Work out the finished part from the listing and answer in its coordinate system (mm). A direction names the side the tool comes from. Give positions to 0.01 mm unless a question says otherwise; leave off trailing zeros. Loops run counter-clockwise (first coordinate to the right, second up) from the corner with the lowest first, then second, coordinate; pieces in that order, holes last. Notation, with made-up numbers: (48, -10) - (61, -10) arc R15 cw to (61, -6) - close; hole circle Ø4 at (49, 73.25). An arc over 180 degrees is marked (long way). One line per question, with ' | ' between items.
from build123d import *

# Parameters (mm, degrees)
F4_DEPTH  = 3.175
F5_DEPTH  = 25.4
F6_R      = 3.1
F6_R_2    = 2.54
F6_W      = 19.05
F6_H      = 3.175
F0_R      = 3.1
F0_R_2    = 1.375
F7_DEPTH  = 3.175
F8_R      = 1.27
F9_DEPTH  = 5.08
F10_R     = 3.048
F11_DEPTH = 3.175
F12_R     = 3.96875
F13_DEPTH = 97.276
F15_DEPTH = 3.175
F16_R     = 2.921
F16_R_2   = 2.54
F17_DEPTH = 3.175
F18_R     = 2.54
F19_R     = 5.08
F19_R_2   = 1.5875
F20_DEPTH = 25.4


with BuildPart() as f4:
    # F3 (on Top) → F4 (new body)
    with BuildSketch(Plane.XY):
        Polygon((-26.1401280605, 113.175), (-34.35, 104.9651280605), (-34.35, -36.6401280605), (-26.1401280605, -44.85), (54.7151280605, -44.85), (62.925, -36.6401280605), (62.925, 104.9651280605), (54.7151280605, 113.175), align=None)
        Polygon((-31.175, 103.65), (-24.825, 110), (53.4, 110), (59.75, 103.65), (59.75, -35.325), (53.4, -41.675), (-24.825, -41.675), (-31.175, -35.325), align=None, mode=Mode.SUBTRACT)
        Polygon((53.4, 110), (-24.825, 110), (-31.175, 103.65), (-31.175, -35.325), (-24.825, -41.675), (53.4, -41.675), (59.75, -35.325), (59.75, 103.65), align=None)
    extrude(amount=-F4_DEPTH)

    # F3 (on Top) → F5 (join)
    with BuildSketch(Plane.XY):
        Polygon((-26.1401280605, 113.175), (-34.35, 104.9651280605), (-34.35, -36.6401280605), (-26.1401280605, -44.85), (54.7151280605, -44.85), (62.925, -36.6401280605), (62.925, 104.9651280605), (54.7151280605, 113.175), align=None)
        Polygon((-31.175, 103.65), (-24.825, 110), (53.4, 110), (59.75, 103.65), (59.75, -35.325), (53.4, -41.675), (-24.825, -41.675), (-31.175, -35.325), align=None, mode=Mode.SUBTRACT)
    extrude(amount=F5_DEPTH)

    # F6 (on face) + F0 (on Top) → F7 (join)
    with BuildSketch(Plane.XY):
        with Locations((-24.5, 23)):
            Circle(F6_R)
        with Locations((24.5, 23)):
            Circle(F6_R)
        with Locations((-24.5, -35)):
            Circle(F6_R)
        with Locations((24.5, -35)):
            Circle(F6_R)
        with Locations((33.715, 43.96)):
            Circle(F6_R_2)
        with Locations((48.955, 43.96)):
            Circle(F6_R_2)
        with Locations((33.715, 22.37)):
            Circle(F6_R_2)
        with Locations((48.955, 22.37)):
            Circle(F6_R_2)
        with Locations((33.715, -0.654)):
            Circle(F6_R_2)
        with Locations((54.035, -0.654)):
            Circle(F6_R_2)
        with Locations((43.875, -30.5625)):
            Rectangle(F6_W, F6_H)
    with BuildSketch(Plane.XY):
        with Locations((-24.5, 23)):
            Circle(F0_R)
        with Locations((-24.5, 23)):
            Circle(F0_R_2, mode=Mode.SUBTRACT)
    extrude(amount=F7_DEPTH)

    # F8 (on face) → F9 (cut)
    with BuildSketch(Plane.XY.offset(3.175)):
        with Locations((-24.5, 23)):
            Circle(F8_R)
        with Locations((24.5, 23)):
            Circle(F8_R)
        with Locations((24.5, -35)):
            Circle(F8_R)
        with Locations((-24.5, -35)):
            Circle(F8_R)
        with Locations((33.715, 43.96)):
            Circle(F8_R)
        with Locations((48.955, 43.96)):
            Circle(F8_R)
        with Locations((33.715, 22.37)):
            Circle(F8_R)
        with Locations((48.955, 22.37)):
            Circle(F8_R)
        with Locations((33.715, -0.654)):
            Circle(F8_R)
        with Locations((54.035, -0.654)):
            Circle(F8_R)
    extrude(amount=-F9_DEPTH, mode=Mode.SUBTRACT)

    # F10 (on face) → F11 (cut, through all)
    with BuildSketch(Plane(origin=(-34.35, 0, 0), x_dir=(0, -1, 0), z_dir=(-1, 0, 0))):
        with Locations((27.2421280605, 19.812)):
            Circle(F10_R)
    extrude(amount=-F11_DEPTH, mode=Mode.SUBTRACT)

    # F12 (on face) → F13 (cut, through all)
    with BuildSketch(Plane(origin=(-34.35, 0, 0), x_dir=(0, -1, 0), z_dir=(-1, 0, 0))):
        with Locations((-94.6463780605, 15.08125)):
            Circle(F12_R)
    extrude(amount=-F13_DEPTH, mode=Mode.SUBTRACT)

    # F14 (on face) → F15 (cut, through all)
    with BuildSketch(Plane(origin=(0, 113.175, 0), x_dir=(-1, 0, 0), z_dir=(0, 1, 0))):
        with BuildLine():
            Line((-19.3675, 20.32), (-20.6375, 20.32))
            ThreePointArc((-20.6375, 20.32), (-21.5355256121, 19.9480256121), (-21.9075, 19.05))
            Line((-21.9075, 19.05), (-21.9075, 6.35))
            ThreePointArc((-21.9075, 6.35), (-21.5355256121, 5.4519743879), (-20.6375, 5.08))
            Line((-20.6375, 5.08), (-19.3675, 5.08))
            ThreePointArc((-19.3675, 5.08), (-18.4694743879, 5.4519743879), (-18.0975, 6.35))
            Line((-18.0975, 6.35), (-18.0975, 19.05))
            ThreePointArc((-18.0975, 19.05), (-18.4694743879, 19.9480256121), (-19.3675, 20.32))
        make_face()
        with BuildLine():
            Line((-25.7175, 6.35), (-25.7175, 19.05))
            ThreePointArc((-25.7175, 19.05), (-26.0894743879, 19.9480256121), (-26.9875, 20.32))
            Line((-26.9875, 20.32), (-28.2575, 20.32))
            ThreePointArc((-28.2575, 20.32), (-29.1555256121, 19.9480256121), (-29.5275, 19.05))
            Line((-29.5275, 19.05), (-29.5275, 6.35))
            ThreePointArc((-29.5275, 6.35), (-29.1555256121, 5.4519743879), (-28.2575, 5.08))
            Line((-28.2575, 5.08), (-26.9875, 5.08))
            ThreePointArc((-26.9875, 5.08), (-26.0894743879, 5.4519743879), (-25.7175, 6.35))
        make_face()
        with BuildLine():
            Line((-33.3375, 6.35), (-33.3375, 19.05))
            ThreePointArc((-33.3375, 19.05), (-33.7094743879, 19.9480256121), (-34.6075, 20.32))
            Line((-34.6075, 20.32), (-35.8775, 20.32))
            ThreePointArc((-35.8775, 20.32), (-36.7755256121, 19.9480256121), (-37.1475, 19.05))
            Line((-37.1475, 19.05), (-37.1475, 6.35))
            ThreePointArc((-37.1475, 6.35), (-36.7755256121, 5.4519743879), (-35.8775, 5.08))
            Line((-35.8775, 5.08), (-34.6075, 5.08))
            ThreePointArc((-34.6075, 5.08), (-33.7094743879, 5.4519743879), (-33.3375, 6.35))
        make_face()
        with BuildLine():
            Line((-40.9575, 6.35), (-40.9575, 19.05))
            ThreePointArc((-40.9575, 19.05), (-41.3294743879, 19.9480256121), (-42.2275, 20.32))
            Line((-42.2275, 20.32), (-43.4975, 20.32))
            ThreePointArc((-43.4975, 20.32), (-44.3955256121, 19.9480256121), (-44.7675, 19.05))
            Line((-44.7675, 19.05), (-44.7675, 6.35))
            ThreePointArc((-44.7675, 6.35), (-44.3955256121, 5.4519743879), (-43.4975, 5.08))
            Line((-43.4975, 5.08), (-42.2275, 5.08))
            ThreePointArc((-42.2275, 5.08), (-41.3294743879, 5.4519743879), (-40.9575, 6.35))
        make_face()
        with BuildLine():
            Line((-7.9375, 19.9480256121), (-9.2075, 19.9480256121))
            ThreePointArc((-9.2075, 19.9480256121), (-10.1055256121, 19.5760512242), (-10.4775, 18.6780256121))
            Line((-10.4775, 18.6780256121), (-10.4775, 6.35))
            ThreePointArc((-10.4775, 6.35), (-10.1055256121, 5.4519743879), (-9.2075, 5.08))
            Line((-9.2075, 5.08), (-7.9375, 5.08))
            ThreePointArc((-7.9375, 5.08), (-7.0394743879, 5.4519743879), (-6.6675, 6.35))
            Line((-6.6675, 6.35), (-6.6675, 18.6780256121))
            ThreePointArc((-6.6675, 18.6780256121), (-7.0394743879, 19.5760512242), (-7.9375, 19.9480256121))
        make_face()
        with BuildLine():
            ThreePointArc((-1.5875, 19.9480256121), (-2.4855256121, 19.5760512242), (-2.8575, 18.6780256121))
            Line((-2.8575, 18.6780256121), (-2.8575, 6.35))
            ThreePointArc((-2.8575, 6.35), (-2.4855256121, 5.4519743879), (-1.5875, 5.08))
            Line((-1.5875, 5.08), (-0.3175, 5.08))
            ThreePointArc((-0.3175, 5.08), (0.5805256121, 5.4519743879), (0.9525, 6.35))
            Line((0.9525, 6.35), (0.9525, 18.6780256121))
            ThreePointArc((0.9525, 18.6780256121), (0.5805256121, 19.5760512242), (-0.3175, 19.9480256121))
            Line((-0.3175, 19.9480256121), (-1.5875, 19.9480256121))
        make_face()
        with BuildLine():
            ThreePointArc((6.0325, 19.9480256121), (5.1344743879, 19.5760512242), (4.7625, 18.6780256121))
            Line((4.7625, 18.6780256121), (4.7625, 6.35))
            ThreePointArc((4.7625, 6.35), (5.1344743879, 5.4519743879), (6.0325, 5.08))
            Line((6.0325, 5.08), (7.3025, 5.08))
            ThreePointArc((7.3025, 5.08), (8.2005256121, 5.4519743879), (8.5725, 6.35))
            Line((8.5725, 6.35), (8.5725, 18.6780256121))
            ThreePointArc((8.5725, 18.6780256121), (8.2005256121, 19.5760512242), (7.3025, 19.9480256121))
            Line((7.3025, 19.9480256121), (6.0325, 19.9480256121))
        make_face()
        with BuildLine():
            ThreePointArc((13.6525, 19.9480256121), (12.7544743879, 19.5760512242), (12.3825, 18.6780256121))
            Line((12.3825, 18.6780256121), (12.3825, 6.35))
            ThreePointArc((12.3825, 6.35), (12.7544743879, 5.4519743879), (13.6525, 5.08))
            Line((13.6525, 5.08), (14.9225, 5.08))
            ThreePointArc((14.9225, 5.08), (15.8205256121, 5.4519743879), (16.1925, 6.35))
            Line((16.1925, 6.35), (16.1925, 18.6780256121))
            ThreePointArc((16.1925, 18.6780256121), (15.8205256121, 19.5760512242), (14.9225, 19.9480256121))
            Line((14.9225, 19.9480256121), (13.6525, 19.9480256121))
        make_face()
    extrude(amount=-F15_DEPTH, mode=Mode.SUBTRACT)

    # F16 (on face) → F17 (cut, through all)
    with BuildSketch(Plane.XZ.offset(44.85)):
        with Locations((-16.8691280605, 19.304)):
            Circle(F16_R)
        with Locations((-4.1691280605, 19.304)):
            Circle(F16_R)
        with Locations((8.5308719395, 19.304)):
            Circle(F16_R)
        with Locations((21.2308719395, 19.304)):
            Circle(F16_R_2)
    extrude(amount=-F17_DEPTH, mode=Mode.SUBTRACT)

    # F18
    f18_edges = [f4.edges().sort_by_distance(p)[0] for p in [
        (62.925, -36.640128, 11.1125),
        (54.715128, -44.85, 11.1125),
        (62.925, 104.965128, 11.1125),
        (54.715128, 113.175, 11.1125),
        (-26.140128, 113.175, 11.1125),
        (-34.35, 104.965128, 11.1125),
        (-34.35, -36.640128, 11.1125),
        (-26.140128, -44.85, 11.1125),
    ]]
    fillet(f18_edges, radius=F18_R)

    # F19 (on face) → F20 (join)
    with BuildSketch(Plane.XY):
        with Locations((-5.775, 89.68)):
            Circle(F19_R)
        with Locations((-5.775, 89.68)):
            Circle(F19_R_2, mode=Mode.SUBTRACT)
        with Locations((29.27, 89.68)):
            Circle(F19_R)
        with Locations((29.27, 89.68)):
            Circle(F19_R_2, mode=Mode.SUBTRACT)
        with Locations((41.97, 10.94)):
            Circle(F19_R)
        with Locations((41.97, 10.94)):
            Circle(F19_R_2, mode=Mode.SUBTRACT)
    extrude(amount=F20_DEPTH)


solid = f4.part
1. Consider L1, parallel to Y at x = 13.5, z = 18 (3 decimals); L2, parallel to X at y = -17, z = 9 (3 decimals); L3, parallel to Y at x = 46.5, z = 17.25 (3 decimals). Determine where each line is inside the solid, lowest interval first.
Evaluation:
L1: -44.85 to -41.675, 110 to 113.175 | L2: -34.35 to -31.175, 59.75 to 62.925 | L3: -44.85 to -41.675, 8.641 to 13.239, 110 to 113.175
2. Find section A-A on y = 66. Write down the section's boundary in (x, z) (3 decimals).
Evaluation:
outline: (-34.35, -3.175) - (62.925, -3.175) - (62.925, 25.4) - (59.75, 25.4) - (59.75, 0) - (-31.175, 0) - (-31.175, 25.4) - (-34.35, 25.4) - close
3. Which of the six approach directions +Z, -Z, +X, -X, +Y, -Y give full straight-line access (tool end or side, diameter ignored) to faces 1 (the cylindrical face through (20.9, -43.285, 21.822)), 2 (the flat face through (21.908, 112, 13)), 3 (the flat face through (34, 24, 3.175))?
Evaluation:
face 1: -Y | face 2: +Y | face 3: +Z
4. Flat-ended cylindrical pins translate along their axes: pin 1 (3 mm diameter, centred on x = 48.955, y = 22.37, fed in from +Z) (3 decimals); pin 2 (3 mm diameter, centred on x = 0.5, y = 36.5, fed in from +Z); pin 3 (1.6 mm diameter, centred on y = 112, z = 10.5, fed in from -X). Find the tip coordinate at first contact, or state that the pin passes through.
Evaluation:
pin 1: z = 3.175 | pin 2: z = 0 | pin 3: x = -28.12
5. Determine the mould class of faces 4 (the flat face through (18.098, 112, 13)), 5 (the flat face through (34, 1, 3.175)), 6 (the cylindrical face through (-24.904, -31.926, 1.565)) for opening direction Z: +Z half, -Z half, draft (parallel to the pull), parting line (faces both ways), or undercut.
Evaluation:
face 4: undercut | face 5: +Z half | face 6: draft
6. Find section B-B on y = 97. Write down the section's boundary in (x, z) (3 decimals).
Evaluation:
outline: (-34.35, -3.175) - (62.925, -3.175) - (62.925, 11.886) - (59.75, 11.886) - (59.75, 0) - (-31.175, 0) - (-31.175, 11.886) - (-34.35, 11.886) - close; (-34.35, 18.277) - (-31.175, 18.277) - (-31.175, 25.4) - (-34.35, 25.4) - close; (59.75, 18.277) - (62.925, 18.277) - (62.925, 25.4) - (59.75, 25.4) - close
